Input: part model. Units: mm. Frame: model coordinates. A direction names the side the tool comes from. Round coordinates to 2 decimals unless told otherwise and drop trailing zeros. Loops run counter-clockwise (first coordinate to the right, second up) from the corner with the lowest first, then second, coordinate; pieces in that order, holes last.
(1) Draft query along Y for faces 1 (the face through (15, 12.75, 2)), 2 (the face through (30, 2.6, 15.5)), 3 (the face through (13.962, 6.204, 1.479)). Return one class per face: released by +Y, released by -Y, zero draft, split by the parting line, or undercut.
(2) Cut plane C-C, the plane x = 15. Output: boundary loops of the cut face in (y, z), and give its area (3 significant figures).
(3) Cut plane D-D, the plane x = 18. Output: boundary loops of the cut face in (y, z).
(4) Line query: line 1 (X direction, y = 0.95, z = 15); line 2 (Z direction, x = 25, y = 1); line 3 (Y direction, x = 14.25, z = 33). Output: solid intervals per line, ascending.
(5) Cut plane B-B, the plane x = 25. Output: boundary loops of the cut face in (y, z), and give its area (3 significant figures).
(6) First-contact query: pin 1 Ø1.5 at (x, y) = (16, 10.5) entering from +Z; pin 2 Ø9 at (x, z) = (21, 21.5) entering from +Y; pin 3 Ø1.5 at (x, z) = (5, 35) entering from +Y. Flat tips, straight axial feed; report the tip coordinate or a pass-through.
(7) Access query for faces 4 (the face through (5.16, 1.48, 33.76)), 5 (the face through (15, 11, 3)). Directions: +Z, -Z, +X, -X, +Y, -Y. A direction counts if a zero-diameter tool reaches every point of the face in a straight line with its end or side. Return the directions, or none.
(8) Cut plane A-A, the plane z = 15. Output: boundary loops of the cut face in (x, y).
from build123d import *

# Parameters (mm, degrees)
T_LE_DE_BASE_PLI_E1_DEPTH = 30
TROU_TARAUD_M31_D         = 2.5
D_GAGEMENT_M41_D          = 4.5


# Sheet-metal steps are written as plain solids
with BuildPart() as part:
    # Esquisse1 → Tôle de base pliée1 (new body)
    with BuildSketch(Plane(origin=(0, 0, 0), x_dir=(0, 0, -1), z_dir=(1, 0, 0))):
        with BuildLine():
            Line((0, 12.75), (0, 4))
            ThreePointArc((0, 4), (-1.171572875, 1.171572875), (-4, 0))
            Line((-4, 0), (-40, 0))
            Line((-40, 0), (-40, 3))
            Line((-40, 3), (-4, 3))
            ThreePointArc((-4, 3), (-3.292893219, 3.292893219), (-3, 4))
            Line((-3, 4), (-3, 12.75))
            Line((-3, 12.75), (0, 12.75))
        make_face()
    extrude(amount=T_LE_DE_BASE_PLI_E1_DEPTH)

    # Trou taraudé M31 (through all)
    with Locations(Plane(origin=(0, 3, 0), x_dir=(1, 0, 0), z_dir=(0, 1, 0))):
        with Locations((5, -35), (5, -15), (25, -15), (25, -35)):
            Hole(TROU_TARAUD_M31_D / 2)

    # Dégagement M41 (through all)
    with Locations(Plane.XY.offset(3)):
        with Locations((15, 8.2)):
            Hole(D_GAGEMENT_M41_D / 2)


solid = part.part
Reported:
1. face 1: released by +Y
1. face 2: zero draft
1. face 3: undercut
2. outline: (0, 4) arc R4 ccw to (4, 0) - (5.95, 0) - (5.95, 3) - (4, 3) arc R1 cw to (3, 4) - (3, 40) - (0, 40) - close; (10.45, 0) - (12.75, 0) - (12.75, 3) - (10.45, 3) - close
2. area: 133 mm2
3. outline: (0, 4) arc R4 ccw to (4, 0) - (12.75, 0) - (12.75, 3) - (4, 3) arc R1 cw to (3, 4) - (3, 40) - (0, 40) - close
4. line 1: x = 0 to 3.75, 6.25 to 23.75, 26.25 to 30
4. line 2: z = 1.35 to 13.75, 16.25 to 33.75, 36.25 to 40
4. line 3: y = 0 to 3
5. outline: (0, 4) arc R4 ccw to (4, 0) - (12.75, 0) - (12.75, 3) - (4, 3) arc R1 cw to (3, 4) - (3, 13.75) - (0, 13.75) - close; (0, 16.25) - (3, 16.25) - (3, 33.75) - (0, 33.75) - close; (0, 36.25) - (3, 36.25) - (3, 40) - (0, 40) - close
5. area: 131 mm2
6. pin 1: stops at z = 3
6. pin 2: stops at y = 3
6. pin 3: passes through
7. face 4: +Y, -Y
7. face 5: +Z, +X, -X, +Y
8. outline: (0, 0) - (3.75, 0) - (3.75, 3) - (0, 3) - close; (6.25, 0) - (23.75, 0) - (23.75, 3) - (6.25, 3) - close; (26.25, 0) - (30, 0) - (30, 3) - (26.25, 3) - close
